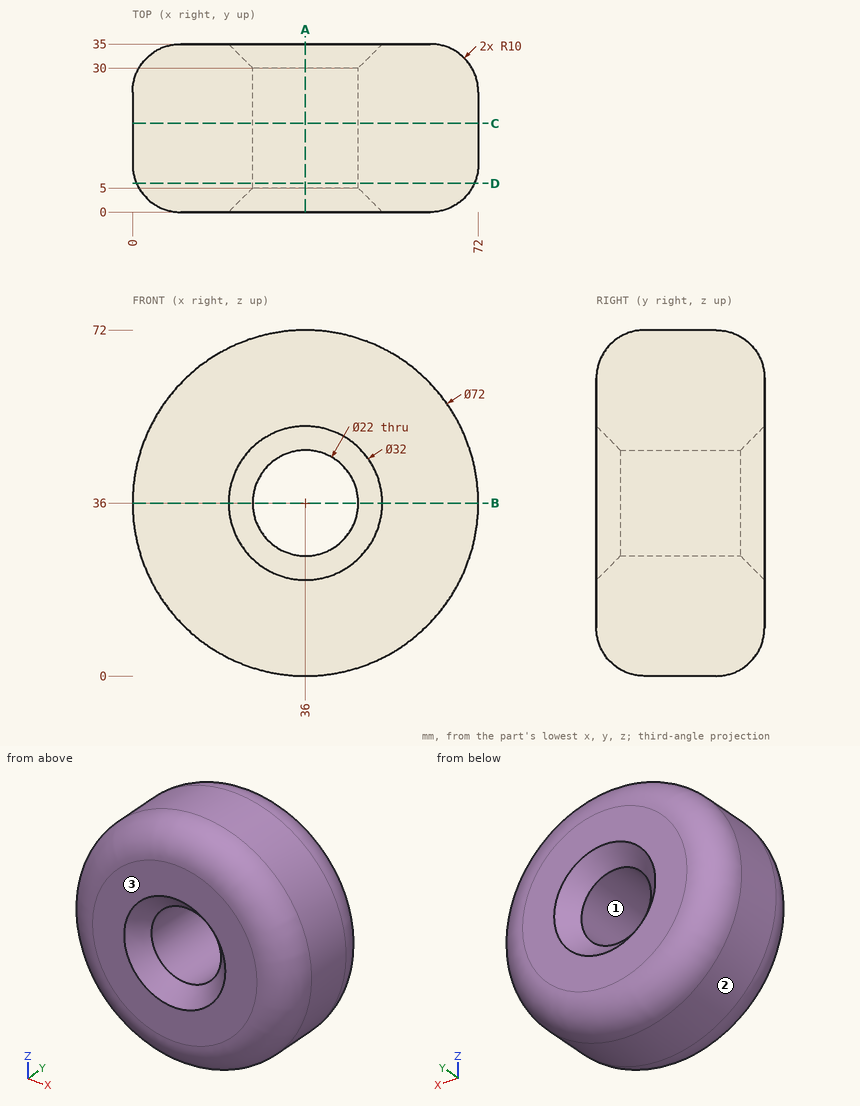
Here's the drawing with two shaded views (mm, measured from the low corner). I have some questions. Coordinates: 2 decimals unless noted, no trailing zeros. Order: outer loops, then holes, each group sorted by start corner. A loop starts at its lowest first (then second) coordinate and runs counter-clockwise, first axis right, second up.
Q1. Will these pins go through, and if not, where does the flat tip stop? pin 1 (1.5 mm diameter, centred on x = 54, z = 50, fed in from -Y); pin 2 (2 mm diameter, centred on x = 29.5, z = 47, fed in from -Y); pin 3 (4 mm diameter, centred on x = 12.5, z = 52.5, fed in from +Y); pin 4 (8 mm diameter, centred on x = 47.5, y = 5, fed in from +Z).
Q2. Thinking about a two-plate mould opening in X: for the marked faces 1, 2 and 3, which applies, released by +X, released by -X, zero draft, split by the parting line, or undercut?
Q3. Please list where these lines run through material, in increasing order: L1, parallel to Z at x = 36, y = 12; L2, parallel to Z at x = 40.5, y = 25; L3, parallel to X at y = 3, z = 31.5.
Q4. Suppose I cut it at D-D on y = 6. Please give me the cut outline in (x, z).
Q5. Suppose I cut it at A-A on x = 36. Please give me the cut outline in (y, z).
Q6. Suppose I cut it at C-C on y = 18.5. Please give me the cut outline in (x, z), and give its area (3 significant figures).
Q7. Suppose I cut it at B-B on z = 36. Please give me the cut outline in (x, y), and give its area (3 significant figures).
Answer:
1. pin 1: stops at y = 0
1. pin 2: stops at y = 2.22
1. pin 3: stops at y = 34.97
1. pin 4: stops at z = 70.69
2. face 1: undercut
2. face 2: split by the parting line
2. face 3: zero draft
3. L1: z = 0 to 25, 47 to 72
3. L2: z = 0.28 to 25.96, 46.04 to 71.72
3. L3: x = 3.17 to 23.8, 48.2 to 68.83
4. outline: circle Ø70.33 at (36, 36); hole circle Ø22 at (36, 36)
5. outline: (0, 10) arc R10 ccw to (10, 0) - (25, 0) arc R10 ccw to (35, 10) - (35, 20) - (30, 25) - (5, 25) - (0, 20) - close; (0, 52) - (5, 47) - (30, 47) - (35, 52) - (35, 62) arc R10 ccw to (25, 72) - (10, 72) arc R10 ccw to (0, 62) - close
6. outline: circle Ø72 at (36, 36); hole circle Ø22 at (36, 36)
6. area: 3,690 mm2
7. outline: (0, 10) arc R10 ccw to (10, 0) - (20, 0) - (25, 5) - (25, 30) - (20, 35) - (10, 35) arc R10 ccw to (0, 25) - close; (47, 5) - (52, 0) - (62, 0) arc R10 ccw to (72, 10) - (72, 25) arc R10 ccw to (62, 35) - (52, 35) - (47, 30) - close
7. area: 1,610 mm2
